Geometry: final body of the model. Coordinates: model frame, mm. Face numbers are marked on the shaded views. A direction names the side the tool comes from. Give positions to 0.01 mm unless a question says otherwise; leave off trailing zeros. Order: outer loops, then holes, each group sorted by start corner. A loop starts at its lowest first (then second) coordinate and runs counter-clockwise, first axis right, second up. Notation, with made-up numbers: (48.5, -15) - (73.5, -15) arc R17 ccw to (73.5, 1) - close; hole circle Ø6 at (69.25, -18.75). An arc over 180 degrees is marked (long way). One line per item, written item: value.
```python
from build123d import *

# Parameters (mm, degrees)
CROQUIS1_W              = 30
CROQUIS1_H              = 24
CROQUIS1_W_2            = 22
CROQUIS1_H_2            = 23
SALIENTE_EXTRUIR1_DEPTH = 15
CROQUIS2_R              = 8.5
CORTAR_EXTRUIR1_DEPTH   = 25
REDONDEO1_R             = 10
REDONDEO2_R             = 10
CROQUIS5_R              = 1.5
CORTAR_EXTRUIR3_DEPTH   = 30
REDONDEO3_R             = 2
CORTAR_EXTRUIR4_DEPTH   = 25
CROQUIS7_R              = 1.25
CORTAR_EXTRUIR5_DEPTH   = 10
REDONDEO4_START         = 1.500000102
REDONDEO4_DEPTH         = 13.499999898
REDONDEO4_START_2       = -11.985627603
REDONDEO4_2_DEPTH       = 10.485627421
REDONDEO4_START_3       = -14.797959071
REDONDEO4_3_DEPTH       = 16.297959173
REDONDEO4_START_4       = -16
REDONDEO4_4_DEPTH       = 4


with BuildPart() as part:
    # Croquis1 → Saliente-Extruir1 (new, symmetric)
    with BuildSketch(Plane.XY):
        Rectangle(CROQUIS1_W, CROQUIS1_H)
        with Locations((-4, -23.5)):
            Rectangle(CROQUIS1_W_2, CROQUIS1_H_2)
    extrude(amount=SALIENTE_EXTRUIR1_DEPTH, both=True)

    # Croquis2 → Cortar-Extruir1 (cut)
    with BuildSketch(Plane(origin=(15, 0, 0), x_dir=(0, 0, -1), z_dir=(1, 0, 0))):
        Circle(CROQUIS2_R)
    extrude(amount=-CORTAR_EXTRUIR1_DEPTH, mode=Mode.SUBTRACT)

    # Redondeo1
    redondeo1_edges = [part.edges().sort_by_distance(p)[0] for p in [
        (-15, 12, 0),
    ]]
    fillet(redondeo1_edges, radius=REDONDEO1_R)

    # Redondeo2
    # the kernel refuses this fillet: 10 mm, written as the material it takes off along each edge
    with BuildSketch(Plane(origin=(15, -37, -15), x_dir=(0, 0, 1), z_dir=(0, 1, 0))) as redondeo2_piece_1:
        with BuildLine():
            CenterArc((REDONDEO2_R, -REDONDEO2_R), REDONDEO2_R, 90, 90)
            Line((0, -REDONDEO2_R), (0, 0))
            Line((0, 0), (REDONDEO2_R, 0))
        make_face()
    extrude(amount=74, mode=Mode.SUBTRACT)

    # Croquis5 → Cortar-Extruir3 (cut)
    with BuildSketch(Plane(origin=(0, 12, 0), x_dir=(1, 0, 0), z_dir=(0, 1, 0))):
        with Locations(Location((10, 0, 0), (0, 0, 270))):
            Circle(CROQUIS5_R)
    extrude(amount=-CORTAR_EXTRUIR3_DEPTH, mode=Mode.SUBTRACT)

    # Redondeo3
    redondeo3_edges = [part.edges().sort_by_distance(p)[0] for p in [
        (15, 0, 15),
    ]]
    fillet(redondeo3_edges, radius=REDONDEO3_R)

    # Croquis6 → Cortar-Extruir4 (cut)
    with BuildSketch(Plane.ZY.offset(15)):
        Polygon((12.5, -32.5), (10, -35), (15, -35), align=None)
        Polygon((7.5, -32.5), (5, -35), (10, -35), align=None)
        Polygon((2.5, -32.5), (0, -35), (5, -35), align=None)
        Polygon((-2.5, -32.5), (-5, -35), (0, -35), align=None)
        Polygon((-7.5, -32.5), (-10, -35), (-5, -35), align=None)
        Polygon((-12.5, -32.5), (-15, -35), (-10, -35), align=None)
    extrude(amount=-CORTAR_EXTRUIR4_DEPTH, mode=Mode.SUBTRACT)

    # Croquis7 → Cortar-Extruir5 (cut)
    with BuildSketch(Plane.ZY.offset(15)):
        with Locations((0, -14)):
            Circle(CROQUIS7_R)
        with Locations((0, -26)):
            Circle(CROQUIS7_R)
    extrude(amount=-CORTAR_EXTRUIR5_DEPTH, mode=Mode.SUBTRACT)

    # Redondeo4: read off the stored shape, not the designer's step
    # Redondeo4 outline → Redondeo4 (add)
    with BuildSketch(Plane.XY.offset(REDONDEO4_START)):
        with BuildLine():
            Line((7, -12), (7, -15))
            ThreePointArc((7, -15), (7.878679656, -12.878679656), (10, -12))
            Line((10, -12), (7, -12))
        make_face()
    extrude(amount=REDONDEO4_DEPTH)

    # Redondeo4 2 outline → Redondeo4 2 (add)
    with BuildSketch(Plane.XY.offset(REDONDEO4_START_2)):
        with BuildLine():
            Line((7, -12), (7, -15))
            ThreePointArc((7, -15), (7.878679656, -12.878679656), (10, -12))
            Line((10, -12), (7, -12))
        make_face()
    extrude(amount=REDONDEO4_2_DEPTH)

    # Redondeo4 3 outline → Redondeo4 3 (add)
    with BuildSketch(Plane.XY.offset(REDONDEO4_START_3)):
        with BuildLine():
            Line((7, -12), (7, -15))
            ThreePointArc((7, -15), (7.878679656, -12.878679656), (10, -12))
            Line((10, -12), (7, -12))
        make_face()
    extrude(amount=REDONDEO4_3_DEPTH)

    # Redondeo4 4 outline → Redondeo4 4 (cut)
    with BuildSketch(Plane(origin=(0, 0, 0), x_dir=(1, 0, 0), z_dir=(0, 1, 0)).offset(REDONDEO4_START_4)):
        with BuildLine():
            ThreePointArc((7, 14.797958971), (8.545926272, 14.350208921), (10, 13.660254038))
            Line((10, 13.660254038), (10, 14.797959071))
            Line((10, 14.797959071), (7, 14.797958971))
        make_face()
        with BuildLine():
            Line((10, -1.5), (10, 1.5))
            ThreePointArc((10, 1.5), (8.5, 0), (10, -1.5))
        make_face()
    extrude(amount=REDONDEO4_4_DEPTH, mode=Mode.SUBTRACT)


solid = part.part
```
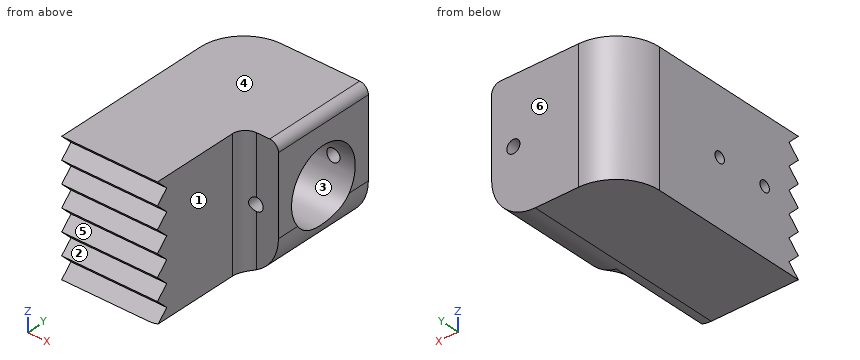
1) Section D-D, the plane x = -9. Return loops of the section in (y, z).
Answers below:
outline: (-35, -15) - (11.17, -15) - (11.17, 15) - (-35, 15) - (-32.5, 12.5) - (-35, 10) - (-32.5, 7.5) - (-35, 5) - (-32.5, 2.5) - (-35, 0) - (-32.5, -2.5) - (-35, -5) - (-32.5, -7.5) - (-35, -10) - (-32.5, -12.5) - close; hole circle Ø2.5 at (-26, 0); hole circle Ø2.5 at (-14, 0); hole circle Ø17 at (0, 0)
2) First-contact query: pin 1 (2 mm diameter, centred on y = -26, z = 0, fed in from -X); pin 2 (2 mm diameter, centred on y = -26, z = 0, fed in from +X); pin 3 (1.5 mm diameter, centred on x = 8, y = -8, fed in from -Z); pin 4 (3.5 mm diameter, centred on x = 10, z = 0, fed in from +Y). Flat tips, straight axial feed; report the tip coordinate or a pass-through.
Answers below:
pin 1: x = -5
pin 2: x = 7
pin 3: z = -14.74
pin 4: y = 12
3) Section B-B, the plane y = -10.5. Return loops of the section in (x, z), then the cut area to 3 significant figures.
Answers below:
outline: (-15, -15) - (5, -15) arc R10 ccw to (15, -5) - (15, 13) arc R2 ccw to (13, 15) - (-15, 15) - close; hole circle Ø3 at (10, 0)
area: 871 mm^2
4) Material intervals for line 1 along X through (y, z) = (-11.5, 0); line 2 along Z through (x, y) = (10, 9.85); line 3 along X through (y, z) = (-15.5, -9), sorted ascending.
Answers below:
line 1: -15 to 8.5, 11.5 to 15
line 2: -13.66 to -1.5, 1.5 to 15
line 3: -15 to 7
5) Set-up query: the marked faces 1, 2 and 3. Return all of +Z, -Z, +X, -X, +Y, -Y with unobstructed straight access to the full face (end or side cutting, diameter ignored); none if empty.
Answers below:
face 1: +Z, -Z, +X, -Y
face 2: +X, -X, -Y
face 3: +X
6) Mould query, pull axis Z, two halves, no side actions, for the marked faces 4, 5 and 6. Classes: released by +Z, released by -Z, zero draft, split by the parting line, or undercut.
Answers below:
face 4: released by +Z
face 5: undercut
face 6: zero draft
7) Section A-A, the plane x = 0.5. Return loops of the section in (y, z), then the cut area to 3 significant figures.
Answers below:
outline: (-35, -15) - (12, -15) - (12, 15) - (-35, 15) - (-32.5, 12.5) - (-35, 10) - (-32.5, 7.5) - (-35, 5) - (-32.5, 2.5) - (-35, 0) - (-32.5, -2.5) - (-35, -5) - (-32.5, -7.5) - (-35, -10) - (-32.5, -12.5) - close; hole circle Ø17 at (0, 0)
area: 1,150 mm^2
8) Section C-C, the plane y = -26. Return loops of the section in (x, z), then the cut area to 3 significant figures.
Answers below:
outline: (-15, -15) - (5, -15) arc R10 ccw to (7, -14.8) - (7, 15) - (-15, 15) - (-15, 1.25) - (-5, 1.25) - (-5, -1.25) - (-15, -1.25) - close
area: 635 mm^2
